Part model, mm, in its own coordinate system. A direction names the side the tool comes from. Coordinates: 2 decimals unless noted, no trailing zeros. Loops run counter-clockwise (first coordinate to the right, second up) from the corner with the lowest first, then second, coordinate; pieces in that order, holes last. Notation, with made-up numbers: (12.5, 38.5) -> (26.5, 38.5) arc R6 cw to (26.5, 44.5) -> close; hole circle Ø4 at (-30, -38.75). An arc over 180 degrees is marked (long way). One line per item, written item: value. Start each with the question number.
from build123d import *

# Parameters (mm, degrees)
SKETCH1_W           = 120
SKETCH1_H           = 150
BOSS_EXTRUDE1_DEPTH = 100
SHELL1_T            = -10
SKETCH2_W           = 10
SKETCH2_H           = 8
BOSS_EXTRUDE2_DEPTH = 10
SKETCH3_R           = 3
CUT_EXTRUDE1_DEPTH  = 206.243757518
FILLET1_R           = 2


with BuildPart() as part:
    # Sketch1 → Boss-Extrude1 (new body)
    with BuildSketch(Plane.XY):
        with Locations((60, 75)):
            Rectangle(SKETCH1_W, SKETCH1_H)
    extrude(amount=BOSS_EXTRUDE1_DEPTH)

    # Shell1
    shell1_openings = [part.faces().sort_by_distance(p)[0] for p in [
        (60, 75, 100),
    ]]
    offset(amount=SHELL1_T, openings=shell1_openings, kind=Kind.INTERSECTION)

    # Sketch2 → Boss-Extrude2 (add)
    with BuildSketch(Plane.XY.offset(100)):
        with Locations((5, 101)):
            Rectangle(SKETCH2_W, SKETCH2_H)
        with Locations((5, 121)):
            Rectangle(SKETCH2_W, SKETCH2_H)
        with Locations((5, 29)):
            Rectangle(SKETCH2_W, SKETCH2_H)
        with Locations((5, 49)):
            Rectangle(SKETCH2_W, SKETCH2_H)
    extrude(amount=BOSS_EXTRUDE2_DEPTH)

    # Sketch3 → Cut-Extrude1 (cut, through all)
    with BuildSketch(Plane(origin=(0, 125, 0), x_dir=(1, 0, 0), z_dir=(0, 1, 0))):
        with Locations(Location((5, -105, 0), (0, 0, 270))):
            Circle(SKETCH3_R)
    extrude(amount=-CUT_EXTRUDE1_DEPTH, mode=Mode.SUBTRACT)

    # Fillet1
    fillet1_edges = [part.edges().sort_by_distance(p)[0] for p in [
        (0, 150, 50),
        (120, 150, 50),
        (120, 0, 50),
        (0, 0, 50),
    ]]
    fillet(fillet1_edges, radius=FILLET1_R)


solid = part.part
1) Slice it at A-A (z = 105). State how many separate pieces and enclosed holes the cut face has, then the cut area to 3 significant figures.
2) Probe line 1 (Y direction, x = 59.5, z = 56.5); line 2 (X direction, y = 35, z = 19.5); line 3 (X direction, y = 103.25, z = 105). List the from-to ranges inside material, lowest first. Write a range as from..to.
3) Pin check, flat tips, straight feed: pin 1 Ø8 at (x, z) = (5, 105) entering from -Y; pin 2 Ø11 at (x, y) = (6.5, 76.5) entering from +Z; pin 3 Ø12 at (x, y) = (45.5, 53) entering from +Z. Stop position of each tip, or through.
4) Slice it at B-B (y = 94.5). Give the cut face in (x, z).
5) Pull direction X, two halves, no side cores. Call faces 1 (the flat face through (59, 76, 10)), 2 (the flat face through (120, 74, 49)), 3 (the flat face through (10, 74, 59)), 4 (the flat face through (5, 121, 110)): +X half, -X half, draft (parallel to the pull), parting line (faces both ways), or undercut.
6) Slice it at C-C (x = 80). Give the cut face in (y, z), then the cut area to 3 significant figures.
7) Tool access for faces 5 (the flat face through (2.7, 25, 107.2)), 6 (the flat face through (5, 29, 110)), 7 (the flat face through (59, 10, 54)), 8 (the flat face through (5, 111, 100)), 9 (the flat face through (59, 76, 0)): list every direction of +Z, -Z, +X, -X, +Y, -Y with a clear straight run to the whole face (end or side of a thin tool).
Check sheet entries:
1. separate pieces: 8
1. enclosed holes: 0
1. area: 128 mm^2
2. line 1: y = 0..10, 140..150
2. line 2: x = 0..10, 110..120
2. line 3: x = 0..2, 8..10
3. pin 1: stops at y = 25
3. pin 2: stops at z = 100
3. pin 3: stops at z = 10
4. outline: (0, 0) -> (120, 0) -> (120, 100) -> (110, 100) -> (110, 10) -> (10, 10) -> (10, 100) -> (0, 100) -> close
5. face 1: undercut
5. face 2: +X half
5. face 3: undercut
5. face 4: draft
6. outline: (0, 0) -> (150, 0) -> (150, 100) -> (140, 100) -> (140, 10) -> (10, 10) -> (10, 100) -> (0, 100) -> close
6. area: 3,300 mm^2
7. face 5: +Z, +X, -X, -Y
7. face 6: +Z, +X, -X, +Y, -Y
7. face 7: +Z
7. face 8: +Z, +X, -X
7. face 9: -Z, +X, -X, +Y, -Y
